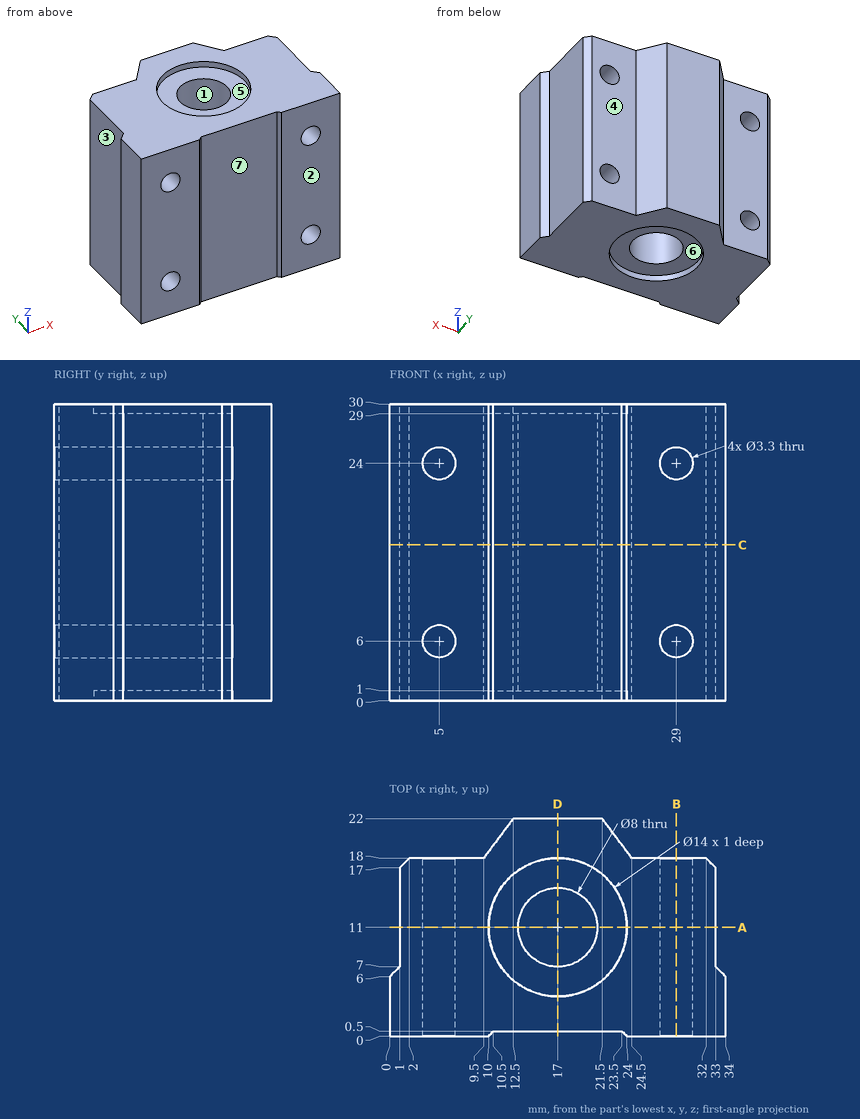
Input: dimensioned drawing with shaded views. Units: mm. Origin: part minimum x, y, z. A direction names the side the tool comes from. Coordinates: 2 decimals unless noted, no trailing zeros. Write each loop counter-clockwise with the first axis right and the second up, starting at its lowest first coordinate (ties: lowest second). Pieces come first, ordered by that corner, then holes. Notation, with made-up numbers: M -27,54 L -19,54 A20 ccw -19,73 Z; hole C 82.25,2.5 d7. An arc over 180 degrees is marked long. Answer as a JSON object with one key per item and string values. Group by question number.
(1) Set-up query: the marked faces 4, 5, 6 and 7. Return all of +Z, -Z, +X, -X, +Y, -Y with unobstructed straight access to the full face (end or side cutting, diameter ignored); none if empty.
(2) Section A-A on y = 11. Output: boundary loops of the cut face in (x, z), plus the area to 3 significant figures.
(3) Mould query, pull axis X, two halves, no side actions, for the marked faces 1, 2 and 3. Classes: pulls with the +X half, pulls with the -X half, needs draft (parallel to the pull), parting line crosses it, or undercut.
(4) Ray query, line 1 along Z through (x, y) = (29, 6.5); line 2 along X through (y, z) = (2.25, 24); line 3 along Y through (x, z) = (17, 22.25). Return the intervals inside material, ascending. Write a range as [from, to].
(5) Section B-B on x = 29. Output: boundary loops of the cut face in (y, z).
(6) Section C-C on z = 15.75. Output: boundary loops of the cut face in (x, y).
(7) Section D-D on x = 17. Output: boundary loops of the cut face in (y, z), plus the area to 3 significant figures.
(8) Contact query for flat-ended pins moving along their axis: P1, Ø2, axis at x = 7.5, z = 12, coming from the +Y side; P2, Ø3, axis at y = 11.5, z = 17.5, coming from the +X side; P3, Ø8, axis at y = 15.5, z = 10, coming from the -X side. Output: stop coordinate, or through.
Result set:
{
 "1": {"face 4": "+Z, -Z, +X, +Y", "face 5": "+Z", "face 6": "-Z", "face 7": "+Z, -Z, -Y"},
 "2": {"outline": "M 1,0 L 10,0 L 10,1 L 13,1 L 13,29 L 10,29 L 10,30 L 1,30 Z; M 21,1 L 24,1 L 24,0 L 33,0 L 33,30 L 24,30 L 24,29 L 21,29 Z; hole C 5,6 d3.3; hole C 5,24 d3.3; hole C 29,6 d3.3; hole C 29,24 d3.3", "area": "674 mm2"},
 "3": {"face 1": "undercut", "face 2": "needs draft", "face 3": "pulls with the -X half"},
 "4": {"line 1": "z = [0, 4.35], [7.65, 22.35], [25.65, 30]", "line 2": "x = [0, 3.35], [6.65, 27.35], [30.65, 34]", "line 3": "y = [0.5, 7], [15, 22]"},
 "5": {"outline": "M 0,0 L 18,0 L 18,4.35 L 0,4.35 Z; M 0,7.65 L 18,7.65 L 18,22.35 L 0,22.35 Z; M 0,25.65 L 18,25.65 L 18,30 L 0,30 Z"},
 "6": {"outline": "M 0,0 L 10,0 L 10.5,0.5 L 23.5,0.5 L 24,0 L 34,0 L 34,6 L 33,7 L 33,17 L 32,18 L 24.5,18 L 21.5,22 L 12.5,22 L 9.5,18 L 2,18 L 1,17 L 1,7 L 0,6 Z; hole C 17,11 d8"},
 "7": {"outline": "M 0.5,0 L 4,0 L 4,1 L 7,1 L 7,29 L 4,29 L 4,30 L 0.5,30 Z; M 15,1 L 18,1 L 18,0 L 22,0 L 22,30 L 18,30 L 18,29 L 15,29 Z", "area": "393 mm2"},
 "8": {"P1": "stops at y = 18", "P2": "stops at x = 33", "P3": "stops at x = 1"}
}
